Verification items for the finished model (mm, model axes). A direction names the side the tool comes from. Round coordinates to 2 decimals unless told otherwise and drop trailing zeros. Order: outer loops, then holes, each group sorted by start corner. A loop starts at its lowest first (then second) coordinate and runs counter-clockwise, first axis right, second up. Notation, with made-up numbers: (-23, -9) -> (26, -9) arc R22 ccw to (26, 24) -> close; hole circle Ø6 at (76.5, 73). An arc over 180 degrees is marked (long way). Put each result on its own line as item: value.
Autodesk Inventor part; units mm, degrees
ref_plane "YZ Plane" through (0, 0, 0) normal (1, 0, 0) x (0, 1, 0)
ref_plane "XZ Plane" through (0, 0, 0) normal (0, 1, 0) x (-1, 0, 0)
ref_plane "XY Plane" through (0, 0, 0) normal (0, 0, 1) x (1, 0, 0)
ref_plane "Arbeitsebene1" through (0, 0, 0) normal (0, 0, 1) x (1, 0, 0)
sketch "Skizze1" plane through (0, 0, 0) normal (0, 0, 1) x (1, 0, 0)
  arc A0 (-34.5, -10.235) -> (-33.9271, -11.9983) centre (-31.5, -10.235) ccw
  line L0 (-21.8951, -28.5589) -> (-33.9271, -11.9983)
  arc A1 (-21.8951, -28.5589) -> (-20.3951, -29.6487) centre (-19.4681, -26.7955) ccw
  line L1 (-0.9271, -35.9742) -> (-20.3951, -29.6487)
  arc A2 (-0.9271, -35.9742) -> (0.9271, -35.9742) centre (0, -33.1211) ccw
  line L2 (20.3951, -29.6487) -> (0.9271, -35.9742)
  arc A3 (20.3951, -29.6487) -> (21.8951, -28.5589) centre (19.4681, -26.7955) ccw
  line L3 (33.9271, -11.9983) -> (21.8951, -28.5589)
  arc A4 (33.9271, -11.9983) -> (34.5, -10.235) centre (31.5, -10.235) ccw
  line L4 (34.5, 10.235) -> (34.5, -10.235)
  arc A5 (34.5, 10.235) -> (33.9271, 11.9983) centre (31.5, 10.235) ccw
  line L5 (21.8951, 28.5589) -> (33.9271, 11.9983)
  arc A6 (21.8951, 28.5589) -> (20.3951, 29.6487) centre (19.4681, 26.7955) ccw
  line L6 (0.9271, 35.9742) -> (20.3951, 29.6487)
  arc A7 (0.9271, 35.9742) -> (-0.9271, 35.9742) centre (0, 33.1211) ccw
  line L7 (-20.3951, 29.6487) -> (-0.9271, 35.9742)
  arc A8 (-20.3951, 29.6487) -> (-21.8951, 28.5589) centre (-19.4681, 26.7955) ccw
  line L8 (-33.9271, 11.9983) -> (-21.8951, 28.5589)
  arc A9 (-33.9271, 11.9983) -> (-34.5, 10.235) centre (-31.5, 10.235) ccw
  line L9 (-34.5, -10.235) -> (-34.5, 10.235)
  circle A10 centre (0, 0) radius 20
  dimension "d0" = 40
extrude "Extrusion1" add sketch "Skizze1" along normal blind 3
ref_plane "Arbeitsebene2" through (-9.734, 3.1628, 3) normal (0.309017, 0.9510565, 0) x (0.9510565, -0.309017, 0)
sketch "Skizze2" plane through (-9.734, 3.1628, 3) normal (0.309017, 0.9510565, 0) x (0.9510565, -0.309017, 0)
  line L0 (46.2092, 3) -> (46.2092, 0)
  line L1 (-25.7393, 3) -> (-25.7393, 0)
  line L2 (30.235, 0) -> (-9.765, 0)
  line L3 (46.2092, 0) -> (20.2284, -15)
  line L4 (46.2092, 0) -> (76.2092, 0) construction
  line L5 (-25.7393, 0) -> (-19.4137, 0)
  line L6 (-25.7393, 0) -> (0.2415, -15)
  line L7 (0.2415, -15) -> (20.2284, -15)
  line L8 (30.235, 0) -> (12.9145, -10)
  line L9 (12.9145, -10) -> (7.5555, -10)
  line L10 (7.5555, -10) -> (-9.765, 0)
  line L11 (-25.7393, 0) -> (-9.765, 0)
  line L12 (30.235, 0) -> (46.2092, 0)
  point P0 (10.235, 3)
  point P1 (-19.4137, 0)
  dimension "d3" = 30
  dimension "d4" = 150
  dimension "d5" = 30
  dimension "d6" = 5
extrude "Extrusion2" add sketch "Skizze2" along normal mid plane 8 contours L12 L3 L7 L6 L5 L11 L10 L9 L8
sketch "Skizze3" plane through (-8.2683, 6.8924, 18) normal (0, 0, 1) x (0.9510565, -0.309017, 0)
  line L0 (44.9692, -8) -> (29.9935, -8)
  line L1 (29.9935, -8) -> (29.9935, -4)
  arc A0 (-10.0065, -4) -> (29.9935, -4) centre (9.9935, -4) ccw
  line L2 (-10.0065, -4) -> (-10.0065, -8)
  line L3 (-10.0065, -8) -> (-24.9823, -8)
  line L4 (-24.9823, -8) -> (-19.6552, -24.3951)
  arc A1 (-19.6552, -24.3951) -> (-18.5654, -25.8951) centre (-16.802, -23.4681) ccw
  line L5 (-18.5654, -25.8951) -> (-2.0049, -37.9271)
  arc A2 (-2.0049, -37.9271) -> (-0.2415, -38.5) centre (-0.2415, -35.5) ccw
  line L6 (-0.2415, -38.5) -> (20.2284, -38.5)
  arc A3 (20.2284, -38.5) -> (21.9918, -37.9271) centre (20.2284, -35.5) ccw
  line L7 (21.9918, -37.9271) -> (38.5523, -25.8951)
  arc A4 (38.5523, -25.8951) -> (39.6421, -24.3951) centre (36.789, -23.4681) ccw
  line L8 (39.6421, -24.3951) -> (44.9692, -8)
  line L9 (44.9692, -8) -> (45.9677, -4.9271)
  line L10 (29.9935, -4) -> (29.9935, 0)
  line L11 (29.9935, 0) -> (44.9692, 0)
  line L12 (44.9692, 0) -> (39.6421, 16.3951)
  arc A5 (39.6421, 16.3951) -> (38.5523, 17.8951) centre (36.789, 15.4681) ccw
  line L13 (38.5523, 17.8951) -> (21.9918, 29.9271)
  arc A6 (21.9918, 29.9271) -> (20.2284, 30.5) centre (20.2284, 27.5) ccw
  line L14 (20.2284, 30.5) -> (-0.2415, 30.5)
  arc A7 (-0.2415, 30.5) -> (-2.0049, 29.9271) centre (-0.2415, 27.5) ccw
  line L15 (-2.0049, 29.9271) -> (-18.5654, 17.8951)
  arc A8 (-18.5654, 17.8951) -> (-19.6552, 16.3951) centre (-16.802, 15.4681) ccw
  line L16 (-19.6552, 16.3951) -> (-24.9823, 0)
  line L17 (-24.9823, 0) -> (-10.0065, 0)
  line L18 (-10.0065, 0) -> (-10.0065, -4)
  arc A9 (29.9935, -4) -> (-10.0065, -4) centre (9.9935, -4) ccw
  line L19 (-24.9823, 0) -> (-25.9808, -3.0729)
  line L20 (-25.9808, -4.9271) -> (-24.9823, -8)
  line L21 (-25.9808, -4.9271) -> (-25.9808, -3.0729)
  line L22 (45.9677, -3.0729) -> (44.9692, 0)
  arc A10 (45.9677, -4.9271) -> (45.9677, -3.0729) centre (43.1145, -4) ccw
  circle A11 centre (9.9935, -4) radius 2.5
  line L23 (0, -8) -> (0, 0)
  line L24 (-25.9808, 0) -> (0, 0)
  line L25 (-25.9808, -3.0729) -> (-25.9808, 0)
  line L26 (-25.9808, -4.9271) -> (-25.9808, -3.0729)
  line L27 (-25.9808, -8) -> (-25.9808, -4.9271)
  line L28 (0, -8) -> (-25.9808, -8)
  line L29 (45.9677, -8) -> (45.9677, -4.9271)
  line L30 (45.9677, -3.0729) -> (45.9677, -4.9271)
  line L31 (45.9677, -3.0729) -> (45.9677, 0)
  line L32 (19.9869, 0) -> (45.9677, 0)
  line L33 (19.9869, -8) -> (19.9869, 0)
  line L34 (45.9677, -8) -> (19.9869, -8)
  point P0 (-24.9823, 0)
  point P1 (-25.9808, -4.9271)
  point P2 (-24.9823, -8)
  point P3 (45.9677, -3.0729)
  point P4 (44.9692, 0)
  point P5 (45.9677, -4.9271)
  point P6 (44.9692, -8)
  dimension "d9" = 5
extrude "Extrusion3" cut sketch "Skizze3" against normal through all contours L9 L29 L34 | L22 L32 L31 | L28 L27 L20 | L19 L25 L24 | A11
fillet "Rundung1" radius 5 4 edges at (9.5044, -3.0882, 18) (-9.5044, 3.0882, 18) (2.5483, -0.828, 13) (-2.5483, 0.828, 13)
properties part number "Anglerfish_Lightplate"
Item 1: Release check for a two-part mould opening along Y. For faces 4 (the cylindrical face through (-4.336, 19.524, 1.479)), 5 (the cylindrical face through (34.35, 11.17, 1.48)), 6 (the cylindrical face through (2.5, 0, 15.5)), 7 (the cylindrical face through (34.357, -11.149, 1.479)) record: +Y half, -Y half, draft (parallel to the pull), parting line (faces both ways), or undercut.
Check sheet entries:
face 4: undercut
face 5: +Y half
face 6: undercut
face 7: -Y half
Item 2: Gauge pin test, flat ends, axial feed: pin 1 Ø0.8 at (x, y) = (1, 3) entering from -Z; pin 2 Ø0.5 at (x, y) = (-34, 11) entering from +Z; pin 3 Ø6 at (x, y) = (1.5, 14.5) entering from +Z; pin 4 Ø4 at (x, y) = (26.5, 20) entering from +Z. Record the tip position at first contact, or that the pin passes through.
Check sheet entries:
pin 1: stops at z = 13
pin 2: stops at z = 3.28
pin 3: passes through
pin 4: stops at z = 3
Item 3: Section check A-A on z = 4.75. Record the boundary of the cut face in (x, y), then the cut area to 3 significant figures.
Check sheet entries:
outline: (-32.57, 6.38) -> (-17.37, 1.44) -> (-14.9, 9.05) -> (-30.09, 13.98) -> close; (14.9, -9.05) -> (30.09, -13.98) -> (32.57, -6.38) -> (17.37, -1.44) -> close
area: 256 mm^2
Item 4: Tool access check on faces 1 (the cylindrical face through (-34.35, -11.17, 1.48)), 2 (the cylindrical face through (-2.771, 0.841, 12.752)), 3 (the flat face through (-1.702, -3.653, 13.728)). Record the directions out of +Z, -Z, +X, -X, +Y, -Y that give a thin tool (end or side, any length) a straight path to the whole face; none if there is none.
Check sheet entries:
face 1: +Z, -Z, -X, -Y
face 2: -Z, -Y
face 3: +Z, -X, -Y
Item 5: Section check C-C on x = 27.5. Record the boundary of the cut face in (y, z).
Check sheet entries:
outline: (-20.84, 0) -> (20.84, 0) -> (20.84, 3) -> (-4.73, 3) -> (-4.73, 7.83) -> (-13.14, 6.33) -> (-13.14, 3) -> (-20.84, 3) -> close
Item 6: Section check B-B on y = -18.5. Record the boundary of the cut face in (x, z).
Check sheet entries:
outline: (-29.2, 0) -> (-7.6, 0) -> (-7.6, 3) -> (-29.2, 3) -> close; (7.6, 0) -> (29.2, 0) -> (29.2, 3) -> (7.6, 3) -> close
Item 7: Material ranges on L1, parallel to Y at x = 0, z = 1.1; L2, parallel to X at y = 0, z = 1.1; L3, parallel to Z at x = 22.5, y = 20.5, recorded low to high. Write a range as [from, to].
Check sheet entries:
L1: y = [-36.12, -20], [20, 36.12]
L2: x = [-34.5, -20], [20, 34.5]
L3: z = [0, 3]
Item 8: Section check D-D on z = 16.5. Record the boundary of the cut face in (x, y).
Check sheet entries:
outline: (-13.21, 0.09) -> (10.74, -7.7) -> (13.21, -0.09) -> (-10.74, 7.7) -> close; hole circle Ø5 at (0, 0)
